Part model, mm, in its own coordinate system. A direction names the side the tool comes from. Give positions to 0.01 mm unless a question says otherwise; leave off trailing zeros. Order: outer loops, then holes, each group sorted by start corner. A loop starts at its lowest first (then second) coordinate and runs counter-clockwise, first axis right, second up. Notation, with made-up numbers: (44, -26.75) - (66, -26.75) arc R27 ccw to (66, -1.75) - close; hole circle Ø10 at (-20.75, -18). An arc over 180 degrees is marked (long way). One line per item, written item: value.
Autodesk Inventor part; units mm, degrees
ref_plane "YZ Plane" through (0, 0, 0) normal (1, 0, 0) x (0, 1, 0)
ref_plane "XZ Plane" through (0, 0, 0) normal (0, 1, 0) x (-1, 0, 0)
ref_plane "XY Plane" through (0, 0, 0) normal (0, 0, 1) x (1, 0, 0)
sketch "Sketch1" plane through (0, 0, 0) normal (0, 0, 1) x (1, 0, 0)
  circle A0 centre (0, 0) radius 4.25
  dimension "d0" = 8.5
extrude "Extrusion1" add sketch "Sketch1" along normal blind 2
sketch "Sketch2" plane through (0, 0, 0) normal (0, 0, -1) x (-1, 0, 0)
  circle A0 centre (0, 0) radius 2.25
  dimension "d3" = 4.5
extrude "Extrusion2" add sketch "Sketch2" along normal blind 8
sketch "Sketch3" plane through (0, 0, 2) normal (0, 0, 1) x (1, 0, 0)
  circle A0 centre (0, 0) radius 2.25
  circle A1 centre (0, 0) radius 4.25
  line L0 (-4.25, 0) -> (-2.125, 3.6806)
  line L1 (-2.125, 3.6806) -> (2.125, 3.6806)
  line L2 (2.125, 3.6806) -> (4.25, 0)
  line L3 (4.25, 0) -> (2.125, -3.6806)
  line L4 (2.125, -3.6806) -> (-2.125, -3.6806)
  line L5 (-2.125, -3.6806) -> (-4.25, 0)
extrude "Extrusion3" add sketch "Sketch3" against normal blind 2 contours L2 A1 | A1 L3 | L1 A1 | A1 L4 | L0 A1 | A1 L5
thread "Thread2"
properties part number "vida"
1) Drill centre lines: line 1 along Z through (x, y) = (-2.5, 3); line 2 along X through (y, z) = (-0.5, -7.5); line 3 along X through (y, z) = (-2.25, 0.5). Where is each one in solid material? Low to high. Write a range as from..to.
Outcome:
line 1: z = 0..2
line 2: x = -2.19..2.19
line 3: x = -3.61..3.61
2) Cut at B-B, the plane z = 0.75. Give the cut face in (x, y).
Outcome:
outline: circle Ø8.5 at (0, 0)
3) Cut at D-D, the plane z = -5.75. Give the cut face in (x, y), then the cut area to 3 significant figures.
Outcome:
outline: circle Ø4.5 at (0, 0)
area: 15.9 mm^2
4) Which spindle directions (+Z, -Z, +X, -X, +Y, -Y) get a long thin tool onto all of the face, cutting with end or side? Do faces 1 (the flat face through (0, 0, 2)), 2 (the cylindrical face through (0.29, -2.23, -3.94)). Say none if no direction does.
Outcome:
face 1: +Z, +X, -X, +Y, -Y
face 2: -Z
5) Cut at A-A, the plane x = 0. Give the cut face in (y, z).
Outcome:
outline: (-4.25, 0) - (-2.25, 0) - (-2.25, -8) - (2.25, -8) - (2.25, 0) - (4.25, 0) - (4.25, 2) - (-4.25, 2) - close
6) Cut at C-C, the plane x = 2. Give the cut face in (y, z), then the cut area to 3 significant figures.
Outcome:
outline: (-3.75, 0) - (-1.03, 0) - (-1.03, -8) - (1.03, -8) - (1.03, 0) - (3.75, 0) - (3.75, 2) - (-3.75, 2) - close
area: 31.5 mm^2
7) Pin check, flat tips, straight feed: pin 1 (2 mm diameter, centred on x = 3, z = -3, fed in from +Y); pin 2 (4 mm diameter, centred on y = -3, z = -1, fed in from -X); pin 3 (1.5 mm diameter, centred on x = 2, z = -1.5, fed in from -Y). Stop position of each tip, or through.
Outcome:
pin 1: stops at y = 1.03
pin 2: stops at x = -4.06
pin 3: stops at y = -1.87
